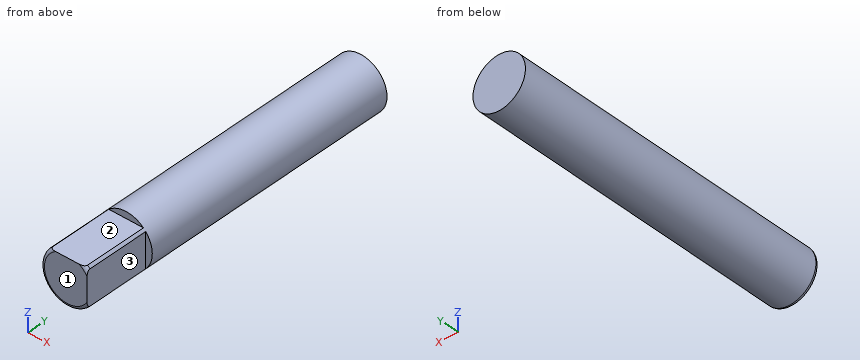
```python
from build123d import *

# Parameters (mm, degrees)
F0_R     = 4
F1_DEPTH = 50
F2_W     = 1
F2_H     = 1
F3_DEPTH = 10
F4_R     = 0.5


with BuildPart() as f1:
    # F0 (on Front) → F1 (new body)
    with BuildSketch(Plane.XZ):
        Circle(F0_R)
    extrude(amount=F1_DEPTH)

    # F2 (on face) → F3 (cut)
    with BuildSketch(Plane.XZ.offset(50)):
        with BuildLine():
            Line((2.6457513111, 3), (3, 3))
            Line((3, 3), (3, 4))
            Line((3, 4), (0, 4))
            ThreePointArc((0, 4), (1.4142135624, 3.7416573868), (2.6457513111, 3))
        make_face()
        with Locations((3.5, 3.5)):
            Rectangle(F2_W, F2_H)
        with BuildLine():
            Line((-4, 3), (-2.6457513111, 3))
            ThreePointArc((-2.6457513111, 3), (-1.4142135624, 3.7416573868), (0, 4))
            Line((0, 4), (-4, 4))
            Line((-4, 4), (-4, 3))
        make_face()
        with BuildLine():
            Line((4, 0), (4, 3))
            Line((4, 3), (3, 3))
            Line((3, 3), (3, 2.6457513111))
            ThreePointArc((3, 2.6457513111), (3.7416573868, 1.4142135624), (4, 0))
        make_face()
        with BuildLine():
            Line((4, -4), (4, 0))
            ThreePointArc((4, 0), (3.7416573868, -1.4142135624), (3, -2.6457513111))
            Line((3, -2.6457513111), (3, -4))
            Line((3, -4), (4, -4))
        make_face()
        with BuildLine():
            Line((-2.6457513111, 3), (2.6457513111, 3))
            ThreePointArc((2.6457513111, 3), (1.4142135624, 3.7416573868), (0, 4))
            ThreePointArc((0, 4), (-1.4142135624, 3.7416573868), (-2.6457513111, 3))
        make_face()
        with BuildLine():
            ThreePointArc((3, -2.6457513111), (3.7416573868, -1.4142135624), (4, 0))
            ThreePointArc((4, 0), (3.7416573868, 1.4142135624), (3, 2.6457513111))
            Line((3, 2.6457513111), (3, -2.6457513111))
        make_face()
    extrude(amount=-F3_DEPTH, mode=Mode.SUBTRACT)

    # F4
    f4_edges = [f1.edges().sort_by_distance(p)[0] for p in [
        (2.828427, -50, 2.828427),
        (-2.828427, -50, -2.828427),
    ]]
    fillet(f4_edges, radius=F4_R)


solid = f1.part
```
Check sheet for the modelled part. Datum: model origin and axes. Units: mm. Face numbers are marked on the shaded views. A direction names the side the tool comes from. Round coordinates to 2 decimals unless told otherwise and drop trailing zeros. Order: outer loops, then holes, each group sorted by start corner. A loop starts at its lowest first (then second) coordinate and runs counter-clockwise, first axis right, second up. Notation, with made-up numbers: M -26,88 L 30,88 A14 cw 30,98 Z; hole C 49,80 d9. An arc over 180 degrees is marked long. Answer in a Markdown table with one row per item.
(1) Material ranges on line 1 along X through (y, z) = (-30.5, 3); line 2 along Y through (x, z) = (3.25, -2); line 3 along Z through (x, y) = (-0.25, -35.5), recorded low to high. Write a range as from..to.
Findings:
| item | result |
|---|---|
| line 1 | x = -2.65..2.65 |
| line 2 | y = -40..0 |
| line 3 | z = -3.99..3.99 |
(2) Section check D-D on y = -15. Record the boundary of the cut face in (x, z).
Findings:
| item | result |
|---|---|
| outline | C 0,0 d8 |
(3) Set-up check for the marked faces 1, 2 and 3: record each of +Z, -Z, +X, -X, +Y, -Y from which the full face is reachable in a straight line by a thin tool's end or side.
Findings:
| item | result |
|---|---|
| face 1 | +Z, -Z, +X, -X, -Y |
| face 2 | +Z, +X, -X, -Y |
| face 3 | +Z, -Z, +X, -Y |
(4) Section check B-B on x = 0. Record the boundary of the cut face in (y, z).
Findings:
| item | result |
|---|---|
| outline | M -50,-3.5 A0.5 ccw -49.5,-4 L 0,-4 L 0,4 L -40,4 L -40,3 L -50,3 Z |
(5) Gauge pin test, flat ends, axial feed: pin 1 (1.6 mm diameter, centred on y = -46.5, z = 0.5, fed in from +X); pin 2 (1 mm diameter, centred on x = 3, y = -17.5, fed in from +Z); pin 3 (2.5 mm diameter, centred on x = 0, y = -43, fed in from +Z). Record the tip position at first contact, or that the pin passes through.
Findings:
| item | result |
|---|---|
| pin 1 | stops at x = 3 |
| pin 2 | stops at z = 3.12 |
| pin 3 | stops at z = 3 |
(6) Section check A-A on z = 0. Record the boundary of the cut face in (x, y), plus the area to 3 significant figures.
Findings:
| item | result |
|---|---|
| outline | M -4,-49.5 A0.5 ccw -3.5,-50 L 3,-50 L 3,-40 L 4,-40 L 4,0 L -4,0 Z |
| area | 390 mm^2 |
